Design review of the part built by this model. Coordinates are the model's own, in mm. Face numbers are marked on the shaded views. A direction names the side the tool comes from. Give positions to 0.01 mm unless a question says otherwise; leave off trailing zeros. Loops run counter-clockwise (first coordinate to the right, second up) from the corner with the lowest first, then second, coordinate; pieces in that order, holes last.
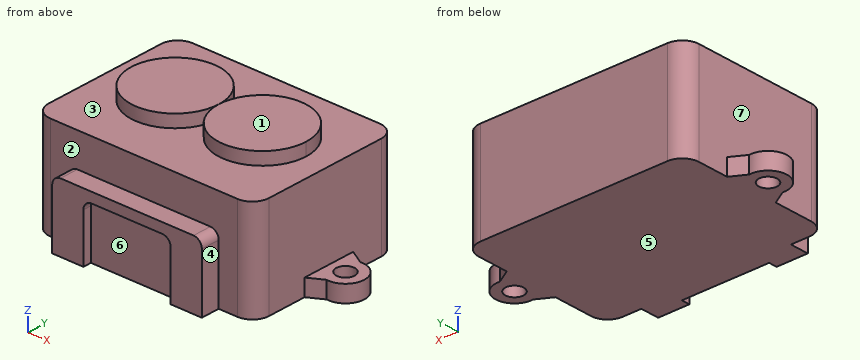
Autodesk Inventor part; units mm, degrees
ref_plane "YZ Plane" through (0, 0, 0) normal (1, 0, 0) x (0, 1, 0)
ref_plane "XZ Plane" through (0, 0, 0) normal (0, 1, 0) x (-1, 0, 0)
ref_plane "XY Plane" through (0, 0, 0) normal (0, 0, 1) x (1, 0, 0)
sketch "Sketch1" plane through (0, 0, 0) normal (0, 0, 1) x (1, 0, 0)
  line L0 (2, 0) -> (24.5, 0)
  line L1 (26.5, 2) -> (26.5, 17)
  line L2 (24.5, 19) -> (2, 19)
  line L3 (0, 17) -> (0, 2)
  arc A0 (2, 19) -> (0, 17) centre (2, 17) ccw
  arc A1 (26.5, 17) -> (24.5, 19) centre (24.5, 17) ccw
  arc A2 (0, 2) -> (2, 0) centre (2, 2) ccw
  arc A3 (24.5, 0) -> (26.5, 2) centre (24.5, 2) ccw
  line L4 (4.25, 0) -> (22.25, 0)
  line L5 (22.25, 0) -> (22.25, -2.25)
  line L6 (22.25, -2.25) -> (4.25, -2.25)
  line L7 (4.25, -2.25) -> (4.25, 0)
  circle A4 centre (-2, 10) radius 1.1
  circle A5 centre (28.5, 10) radius 1.1
  arc A6 (-1.7552, 12.2366) -> (-1.7552, 7.7634) centre (-2, 10) ccw
  arc A7 (28.2552, 7.7634) -> (28.2552, 12.2366) centre (28.5, 10) ccw
  circle A8 centre (18.5, 10) radius 5.25
  circle A9 centre (8, 10) radius 5.25
  line L8 (-1.7552, 12.2366) -> (0, 13.25)
  line L9 (-1.7552, 7.7634) -> (0, 6.75)
  line L10 (13.25, 19) -> (13.25, 0) construction
  line L11 (28.2552, 12.2366) -> (26.5, 13.25)
  line L12 (28.2552, 7.7634) -> (26.5, 6.75)
  circle A10 centre (8, 10) radius 5
  circle A11 centre (18.5, 10) radius 5
  point P0 (0, 0)
  point P1 (26.5, 19)
  point P2 (26.5, 0)
  point P3 (0, 19)
  point P4 (13.25, 0)
  point P5 (13.25, -2.25)
  point P6 (13.25, 10)
  dimension "d10" = 10.5
  dimension "d11" = 10.5
  dimension "d0" = 26.5
  dimension "d1" = 19
  dimension "d2" = 2
  dimension "d3" = 21.25
  dimension "d4" = 18
  dimension "d5" = 2.2
  dimension "d6" = 4.5
  dimension "d7" = 4.5
  dimension "d8" = 9
  dimension "d9" = 30.5
  dimension "d12" = 10.5
  dimension "d13" = 15.25
  dimension "d14" = 60
  dimension "d15" = 60
  dimension "d16" = 3.25
  dimension "d17" = 3.25
  dimension "d18" = 10
  dimension "d19" = 10
  dimension "d20" = 60
  dimension "d21" = 60
  dimension "d22" = 3.25
  dimension "d23" = 3.25
  dimension "d24" = 10
  dimension "d25" = 10
extrude "Extrusion1" add sketch "Sketch1" along normal blind 12 contours A2 L3 A0 L2 A1 L1 A3 L0
extrude "Extrusion2" add sketch "Sketch1" along normal blind 2 contours L9 A6 L8 L3 | L1 L11 A7 L12
extrude "Extrusion3" add sketch "Sketch1" along normal blind 8 contours L0 L5 L6 L7
fillet "Fillet1" radius 1 2 edges at (4.25, -1.125, 8) (22.25, -1.125, 8)
sketch "Sketch2" plane through (4.25, -2.25, 0) normal (0, -1, 0) x (1, 0, 0)
  line L0 (0, 0) -> (18, 0)
  line L1 (3.75, 0) -> (14.25, 0)
  line L2 (14.25, 0) -> (14.25, 5.8)
  line L3 (13.25, 6.8) -> (4.75, 6.8)
  line L4 (3.75, 5.8) -> (3.75, 0)
  line L5 (1, 8) -> (17, 8)
  arc A0 (4.75, 6.8) -> (3.75, 5.8) centre (4.75, 5.8) ccw
  arc A1 (14.25, 5.8) -> (13.25, 6.8) centre (13.25, 5.8) ccw
  point P0 (-4.25, 0)
  point P1 (9, 6.8)
  point P2 (9, 8)
  dimension "d33" = 6.8
  dimension "d35" = 10.5
  dimension "d36" = 1
extrude "Extrusion4" cut sketch "Sketch2" against normal blind 1
extrude "Extrusion5" add sketch "Sketch1" along normal blind 13.5 contours A8 | A9 | A10 | A11
properties part number "lidarsensor"
Q1. Take a section at C-C (x = 12.5). Give the boundary of the cut face in (y, z).
Results:
outline: (-2.25, 6.8) - (-1.25, 6.8) - (-1.25, 0) - (19, 0) - (19, 12) - (12.7, 12) - (12.7, 13.5) - (7.3, 13.5) - (7.3, 12) - (0, 12) - (0, 8) - (-2.25, 8) - close
Q2. Take a section at A-A (y = 10.75). Give the boundary of the cut face in (x, z), plus the area to 3 significant figures.
Results:
outline: (-4.12, 0) - (-2.8, 0) - (-2.8, 2) - (-4.12, 2) - close; (-1.2, 0) - (27.7, 0) - (27.7, 2) - (26.5, 2) - (26.5, 12) - (23.7, 12) - (23.7, 13.5) - (13.3, 13.5) - (13.3, 12) - (13.2, 12) - (13.2, 13.5) - (2.8, 13.5) - (2.8, 12) - (0, 12) - (0, 2) - (-1.2, 2) - close; (29.3, 0) - (30.62, 0) - (30.62, 2) - (29.3, 2) - close
area: 359 mm2
Q3. Insertion check: pin 1 (1 mm diameter, centred on x = 25.5, y = 4, fed in from +Z); pin 2 (1.1 mm diameter, centred on y = -2, z = 3, fed in from +X); pin 3 (3 mm diameter, centred on x = 11, z = 4.5, fed in from -Y). Each pin has a flat end and moves straight along its axis. Give the tip position at first contact, or say it passes through.
Results:
pin 1: stops at z = 12
pin 2: stops at x = 22.25
pin 3: stops at y = -1.25
Q4. Draft analysis for pull direction X (two halves, no side actions). For the marked faces 5, 6 and 7, state which applies: pulls with the +X half, pulls with the -X half, needs draft (parallel to the pull), parting line crosses it, or undercut.
Results:
face 5: needs draft
face 6: undercut
face 7: pulls with the -X half
Q5. Tool access review of the marked faces 1, 2, 3 and 4: name each direction out of +Z, -Z, +X, -X, +Y, -Y from which nothing blocks a thin tool from reaching the whole face with its end or side.
Results:
face 1: +Z, +X, -X, +Y, -Y
face 2: +Z, -Y
face 3: +Z
face 4: +Z, -Z, +X, -Y
Q6. Wall thickness on line 1 (Y direction, x = -2, z = 0.55); line 2 (Y direction, x = 3.5, z = 6.25); line 3 (Y direction, x = 13, z = 6): over which ranges is each line inside the solid? List them lowest first.
Results:
line 1: y = 7.75 to 8.9, 11.1 to 12.25
line 2: y = 0 to 19
line 3: y = -1.25 to 19
Q7. Take a section at D-D (y = -0.5). Give the boundary of the cut face in (x, z).
Results:
outline: (4.25, 0) - (22.25, 0) - (22.25, 7) arc R1 ccw to (21.25, 8) - (5.25, 8) arc R1 ccw to (4.25, 7) - close
Q8. Take a section at B-B (y = 14.75). Give the boundary of the cut face in (x, z), plus the area to 3 significant figures.
Results:
outline: (0, 0) - (26.5, 0) - (26.5, 12) - (20.74, 12) - (20.74, 13.5) - (16.26, 13.5) - (16.26, 12) - (10.24, 12) - (10.24, 13.5) - (5.76, 13.5) - (5.76, 12) - (0, 12) - close
area: 331 mm2
